```python
from build123d import *

# Parameters (mm, degrees)
SKETCH1_W           = 10
SKETCH1_H           = 30
BOSS_EXTRUDE1_DEPTH = 2
BOSS_EXTRUDE2_DEPTH = 4
SKETCH4_R           = 1
BOSS_EXTRUDE3_DEPTH = 7.5


with BuildPart() as part:
    # Sketch1 → Boss-Extrude1 (new body)
    with BuildSketch(Plane.XY):
        Rectangle(SKETCH1_W, SKETCH1_H)
    extrude(amount=BOSS_EXTRUDE1_DEPTH)

    # Sketch2 → Boss-Extrude2 (add)
    with BuildSketch(Plane.XY.offset(2)):
        Polygon((1, 14), (1, -14), (5, -14), (5, -15), (-5, -15), (-5, -14), (-1, -14), (-1, 14), (-5, 14), (-5, 15), (5, 15), (5, 14), align=None)
    extrude(amount=BOSS_EXTRUDE2_DEPTH)

    # Sketch4 → Boss-Extrude3 (add)
    with BuildSketch(Plane(origin=(0, 0, 0), x_dir=(-1, 0, 0), z_dir=(0, 0, -1))):
        with Locations((0, 2)):
            Circle(SKETCH4_R)
        with Locations((0, -2)):
            Circle(SKETCH4_R)
    extrude(amount=BOSS_EXTRUDE3_DEPTH)


solid = part.part
```
Verification items for the finished model (mm, model axes). A direction names the side the tool comes from. Give positions to 0.01 mm unless a question says otherwise; leave off trailing zeros. Order: outer loops, then holes, each group sorted by start corner. A loop starts at its lowest first (then second) coordinate and runs counter-clockwise, first axis right, second up. Notation, with made-up numbers: M 64,-35 L 84,-35 A26 ccw 84,-12 Z; hole C -7,-40 d2. An arc over 180 degrees is marked long. Return JSON: item names as keys, results as strings. Group by question number.
1) Access from +Z, -Z, +X, -X, +Y, -Y to the whole of each face (thin tool, end or side, straight path). Record for faces 5 (the face through (3, -14, 4)), 6 (the face through (-3, -14, 4)), 7 (the face through (0, -3, -4)).
2) Mould release check, pull along Y, two halves, no side actions. Record for faces 1 (the face through (0, 15, 3)), 2 (the face through (1, 0, 4)), 3 (the face through (-1, 0, 4)), 4 (the face through (0, 2, -7.5)): pulls with the +Y half, pulls with the -Y half, needs draft (parallel to the pull), parting line crosses it, or undercut.
3) Section check D-D on y = -2. Record the cut outline in (x, z), and give its area (3 significant figures).
4) Go/stop test with flat-tipped pins: pin 1 Ø2 at (x, y) = (2.5, 9) entering from +Z; pin 2 Ø3 at (y, z) = (3.5, 4) entering from -X; pin 3 Ø1 at (x, y) = (3.5, -4.5) entering from -Z; pin 4 Ø4 at (x, z) = (4, -5) entering from +Y. Record where each tip stops, or that it passes through.
5) Section check A-A on y = -12.75. Record the cut outline in (x, z), and give its area (3 significant figures).
6) Section check B-B on x = -1.5. Record the cut outline in (y, z), and give its area (3 significant figures).
7) Scan lines: line 1 (Y direction, x = 1.75, z = 2.75); line 2 (Z direction, x = 2.5, y = 5); line 3 (X direction, y = -12, z = 5.5). Record each from-to range of solid material in increasing order.
8) Section check C-C on z = -3.75. Record the cut outline in (x, y).
Answer block:
{
 "1": {"face 5": "+Z, +X", "face 6": "+Z, -X", "face 7": "-Z"},
 "2": {"face 1": "pulls with the +Y half", "face 2": "undercut", "face 3": "undercut", "face 4": "needs draft"},
 "3": {"outline": "M -5,0 L -1,0 L -1,-7.5 L 1,-7.5 L 1,0 L 5,0 L 5,2 L 1,2 L 1,6 L -1,6 L -1,2 L -5,2 Z", "area": "43.0 mm^2"},
 "4": {"pin 1": "stops at z = 2", "pin 2": "stops at x = -1", "pin 3": "stops at z = 0", "pin 4": "passes through"},
 "5": {"outline": "M -5,0 L 5,0 L 5,2 L 1,2 L 1,6 L -1,6 L -1,2 L -5,2 Z", "area": "28.0 mm^2"},
 "6": {"outline": "M -15,0 L 15,0 L 15,6 L 14,6 L 14,2 L -14,2 L -14,6 L -15,6 Z", "area": "68.0 mm^2"},
 "7": {"line 1": "y = -15 to -14, 14 to 15", "line 2": "z = 0 to 2", "line 3": "x = -1 to 1"},
 "8": {"outline": "C 0,-2 d2; C 0,2 d2"}
}
